Source: CAD feature listing. Evaluate the final solid. Frame: model axes, mm. Face numbers are marked on the shaded views. A direction names the side the tool comes from. Give positions to 0.01 mm unless a question says otherwise; leave off trailing zeros. Order: outer loops, then holes, each group sorted by start corner. A loop starts at its lowest first (then second) coordinate and runs counter-clockwise, first axis right, second up.
1) First-contact query: P1, Ø1.2, axis at y = -4, z = 21.5, coming from the +X side; P2, Ø2, axis at y = -4, z = 22, coming from the -X side; P3, Ø1, axis at x = 3, z = 28, coming from the +Y side. Flat tips, straight axial feed; report the tip coordinate or a pass-through.
2) Section A-A, the plane x = 3.5. Return loops of the section in (y, z), plus the area to 3 significant figures.
3) Section B-B, the plane z = 30. Return loops of the section in (x, y).
4) Material intervals for line 1 (Y direction, x = 23, z = 1); line 2 (X direction, y = -2.5, z = 25.5); line 3 (X direction, y = -5.25, z = 24), sorted ascending.
5) Draft query along X for the marked faces 5, 6, 7 and 8. Return one class per face: released by +X, released by -X, zero draft, split by the parting line, or undercut.
6) Access query for the marked faces 1, 2, 3 and 4. Directions: +Z, -Z, +X, -X, +Y, -Y. A direction counts if a zero-diameter tool reaches every point of the face in a straight line with its end or side. Return the directions, or none.
```python
from build123d import *

# Parameters (mm, degrees)
F0_R     = 1
F1_DEPTH = 1.5
F4_DEPTH = 1.5
F5_DEPTH = 5
F3_W     = 4.5
F3_H     = 4.5
F3_R     = 1
F6_DEPTH = 3.5
F7_W     = 32.583123
F7_H     = 2.642157
F8_DEPTH = 14.8


with BuildPart() as f1:
    # F0 (on Top) → F1 (new body)
    with BuildSketch(Plane.XY):
        with BuildLine():
            ThreePointArc((-20.5, 0), (-21.232233, 1.767767), (-23, 2.5))
            ThreePointArc((-23, 2.5), (-25.5, 0), (-23, -2.5))
            ThreePointArc((-23, -2.5), (-21.232233, -1.767767), (-20.5, 0))
        make_face()
        with Locations((-23, 0)):
            Circle(F0_R, mode=Mode.SUBTRACT)
        with BuildLine():
            Line((23, 2.5), (-23, 2.5))
            ThreePointArc((-23, 2.5), (-21.232233, 1.767767), (-20.5, 0))
            ThreePointArc((-20.5, 0), (-21.232233, -1.767767), (-23, -2.5))
            Line((-23, -2.5), (23, -2.5))
            ThreePointArc((23, -2.5), (20.5, 0), (23, 2.5))
        make_face()
        with BuildLine():
            ThreePointArc((25.5, 0), (24.767767, 1.767767), (23, 2.5))
            ThreePointArc((23, 2.5), (20.5, 0), (23, -2.5))
            ThreePointArc((23, -2.5), (24.767767, -1.767767), (25.5, 0))
        make_face()
        with Locations((23, 0)):
            Circle(F0_R, mode=Mode.SUBTRACT)
    extrude(amount=F1_DEPTH)

    # F3 (on face) → F4 (join)
    with BuildSketch(Plane(origin=(0, -2.168101, -0.382295), x_dir=(1, 0, 0), z_dir=(0, -0.984808, -0.173648))):
        Polygon((8.2, 38.13412), (-8.2, 38.13412), (-8.2, 33.63412), (-12.7, 33.63412), (-12.7, 25.68412), (-8.2, 25.68412), (-8.2, 21.18412), (-12.7, 21.18412), (-12.7, 13.73412), (-8.25, 13.73412), (-8.25, 12.23412), (-12.7, 12.23412), (-12.7, 0.43412), (12.7, 0.43412), (12.7, 12.23412), (8.25, 12.23412), (8.25, 13.73412), (12.7, 13.73412), (12.7, 21.18412), (8.2, 21.18412), (8.2, 25.68412), (12.7, 25.68412), (12.7, 33.63412), (8.2, 33.63412), align=None)
        Polygon((-6.5, 27.93412), (-4.5, 27.93412), (4.5, 27.93412), (6.5, 27.93412), (6.5, 16.93412), (-6.5, 16.93412), align=None, mode=Mode.SUBTRACT)
    extrude(amount=-F4_DEPTH)

    # F3 (on face) → F5 (join)
    with BuildSketch(Plane(origin=(0, -2.168101, -0.382295), x_dir=(1, 0, 0), z_dir=(0, -0.984808, -0.173648))):
        Polygon((-12.7, 33.63412), (-12.7, 38.13412), (-8.2, 38.13412), (8.2, 38.13412), (12.7, 38.13412), (12.7, 33.63412), (12.7, 25.68412), (12.7, 21.18412), (12.7, 13.73412), (8.25, 13.73412), (8.25, 12.23412), (12.7, 12.23412), (12.7, 0.43412), (14.2, 0.43412), (14.2, 39.63412), (-14.2, 39.63412), (-14.2, 0.43412), (-12.7, 0.43412), (-12.7, 12.23412), (-8.25, 12.23412), (-8.25, 13.73412), (-12.7, 13.73412), (-12.7, 21.18412), (-12.7, 25.68412), align=None)
    extrude(amount=-F5_DEPTH)

    # F3 (on face) → F6 (join)
    with BuildSketch(Plane(origin=(0, -2.168101, -0.382295), x_dir=(1, 0, 0), z_dir=(0, -0.984808, -0.173648))):
        with Locations((-10.45, 35.88412)):
            Rectangle(F3_W, F3_H)
        with Locations((-10.5, 35.93412)):
            Circle(F3_R, mode=Mode.SUBTRACT)
        with Locations((10.45, 35.88412)):
            Rectangle(F3_W, F3_H)
        with Locations((10.5, 35.93412)):
            Circle(F3_R, mode=Mode.SUBTRACT)
        with Locations((10.45, 23.43412)):
            Rectangle(F3_W, F3_H)
        with Locations((10.5, 23.43412)):
            Circle(F3_R, mode=Mode.SUBTRACT)
        with Locations((-10.45, 23.43412)):
            Rectangle(F3_W, F3_H)
        with Locations((-10.5, 23.43412)):
            Circle(F3_R, mode=Mode.SUBTRACT)
        Polygon((-4.5, 18.93412), (-4.5, 27.93412), (-6.5, 27.93412), (-6.5, 16.93412), (6.5, 16.93412), (6.5, 27.93412), (4.5, 27.93412), (4.5, 18.93412), align=None)
    extrude(amount=-F6_DEPTH)

    # F7 (on face) → F8 (cut)
    with BuildSketch(Plane(origin=(0, 0, 0), x_dir=(1, 0, 0), z_dir=(0, 0, -1))):
        with Locations((-0.506625, -3.821079)):
            Rectangle(F7_W, F7_H)
    extrude(amount=-F8_DEPTH, mode=Mode.SUBTRACT)


solid = f1.part
```
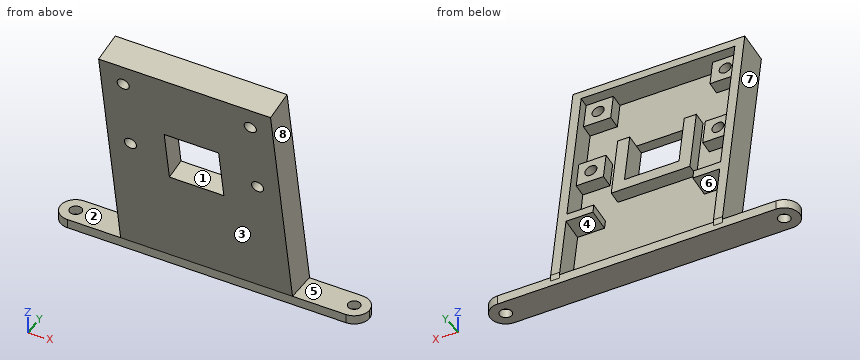
From the geometry:
1. P1: stops at x = 14.2
1. P2: stops at x = -14.2
1. P3: stops at y = -5.56
2. outline: (-9.05, 38.65) - (-7.02, 27.13) - (-5.54, 27.39) - (-7.31, 37.43) - (-3.87, 38.04) - (-4.13, 39.52) - close; (-5.46, 18.26) - (-2.5, 1.5) - (-2.5, 0) - (2.5, 0) - (2.5, 1.5) - (-0.98, 1.5) - (-3.63, 16.56) - (-1.66, 16.9) - (-2.01, 18.87) - close
2. area: 60.0 mm2
3. outline: (-14.2, -7.53) - (14.2, -7.53) - (14.2, -2.45) - (12.7, -2.45) - (12.7, -6) - (-12.7, -6) - (-12.7, -2.45) - (-14.2, -2.45) - close
4. line 1: y = -2.5 to -1, 1 to 2.5
4. line 2: x = -14.2 to -12.7, 12.7 to 14.2
4. line 3: x = -14.2 to -4.5, 4.5 to 14.2
5. face 5: zero draft
5. face 6: undercut
5. face 7: released by -X
5. face 8: released by +X
6. face 1: -Y
6. face 2: +Z, -X, +Y, -Y
6. face 3: -Z, +X, -X, -Y
6. face 4: +Y
